Can you work these out from the drawing? Everything is in mm from the part's minimum corner. A direction names the side the tool comes from. Coordinates: 2 decimals unless noted, no trailing zeros. Order: outer loops, then holes, each group sorted by start corner. A loop starts at its lowest first (then second) coordinate and runs counter-clockwise, first axis right, second up. Notation, with made-up numbers: (26, 12.5) -> (71, 12.5) arc R9 ccw to (71, 18.5) -> close; hole circle Ø7 at (-40, 59). An arc over 180 degrees is marked (long way). Return JSON: item names as keys, results as strings. Group by question number.
1) If we section it at A-A, the plane y = 25.75: State how many separate pieces and enclosed holes the cut face has.
2) If we section it at C-C, the plane x = 31: Please give me the cut outline in (y, z).
3) If we section it at B-B, the plane z = 27: Please give me the cut outline in (x, y).
4) For the marked faces 1, 2 and 3, which set-ups out of +Z, -Z, +X, -X, +Y, -Y let a thin tool reach every point of the face, with its end or its side?
5) If I drill on probe 1 along Z at (x, y) = (30.5, 15.25) (1 decimal); probe 2 along Z at (x, y) = (107, 18.75) (1 decimal), over which ranges is the centre line in solid material (lowest first)? Write a range as from..to.
6) For pin 1 (1 mm diameter, centred on y = 11.5, z = 6, fed in from -X); pin 2 (10 mm diameter, centred on x = 92.5, y = 20, fed in from -Z); pin 3 (1.8 mm diameter, centred on x = 94.2, z = 31.75, fed in from +Y); pin 4 (3 mm diameter, centred on x = 45, y = 17, fed in from -Z) (1 decimal), each with a flat end and sliding along its axis, tell me the tip position at first contact or that it passes through.
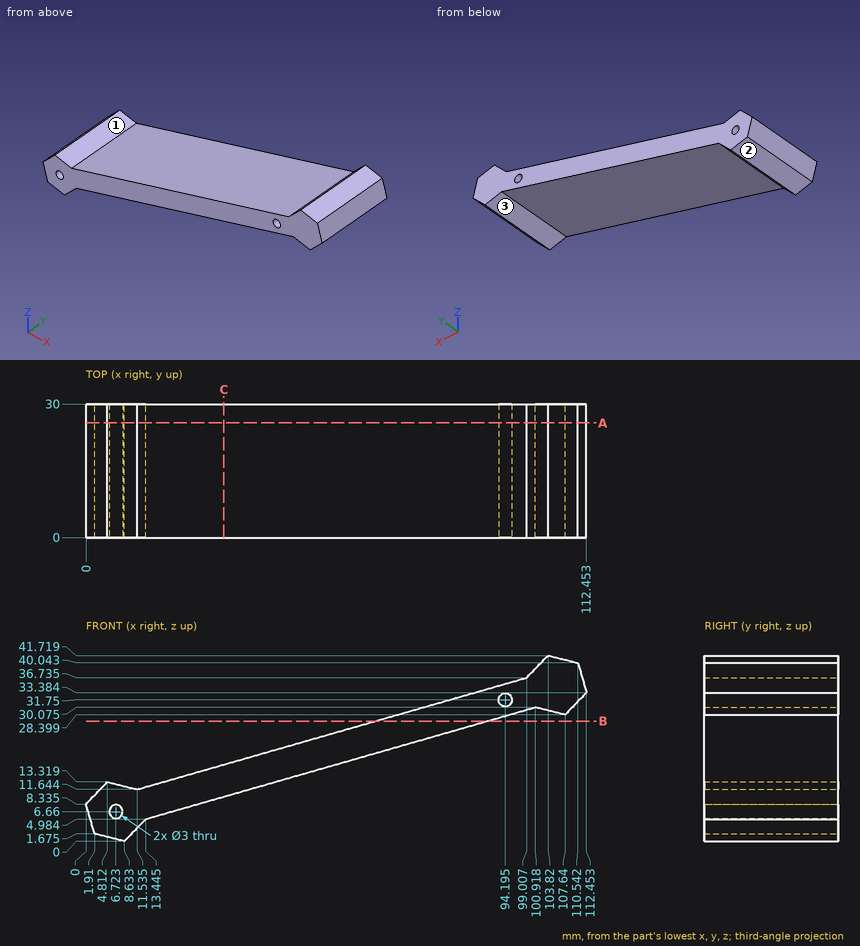
Result sheet:
{
 "1": {"separate pieces": "1", "enclosed holes": "2"},
 "2": {"outline": "(0, 10.02) -> (30, 10.02) -> (30, 17.23) -> (0, 17.23) -> close"},
 "3": {"outline": "(65.07, 0) -> (90.2, 0) -> (90.2, 30) -> (65.07, 30) -> close"},
 "4": {"face 1": "+Z, +Y, -Y", "face 2": "-Z, -X, +Y, -Y", "face 3": "-Z, +Y, -Y"},
 "5": {"probe 1": "z = 9.9..17.1", "probe 2": "z = 28.6..40.9"},
 "6": {"pin 1": "stops at x = 0.53", "pin 2": "stops at z = 26.23", "pin 3": "passes through", "pin 4": "stops at z = 13.6"}
}
